Verification items for this drawing (mm, ordinates from the low corner). Coordinates: 2 decimals unless noted, no trailing zeros. Loops run counter-clockwise (first coordinate to the right, second up) from the corner with the lowest first, then second, coordinate; pieces in that order, holes last. Notation, with made-up numbers: (28, -31.75) -> (59, -31.75) arc R15 cw to (59, -20.75) -> close; hole circle Ø1 at (62, 30). An arc over 180 degrees is marked (long way). Write item = value, one per line.
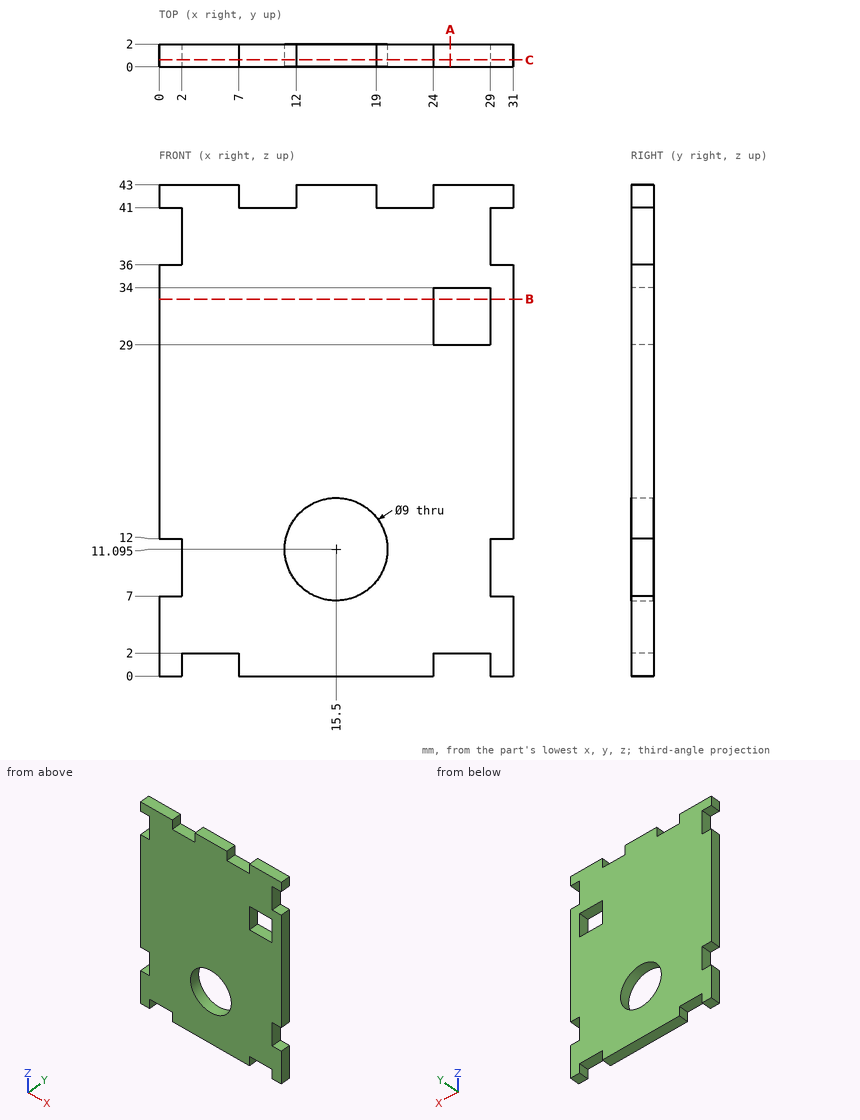
1) Sectioned sample at A-A, the plane x = 25.5. Record the cut outline in (y, z), plus the area to 3 significant figures.
Ans:
outline = (0, 2) -> (2, 2) -> (2, 29) -> (0, 29) -> close; (0, 34) -> (2, 34) -> (2, 43) -> (0, 43) -> close
area = 72.0 mm2
2) Sectioned sample at B-B, the plane z = 33. Record the cut outline in (x, y), plus the area to 3 significant figures.
Ans:
outline = (0, 0) -> (24, 0) -> (24, 2) -> (0, 2) -> close; (29, 0) -> (31, 0) -> (31, 2) -> (29, 2) -> close
area = 52.0 mm2
3) Sectioned sample at C-C, the plane y = 0.6. Count the separate pieces of the cut face and the enclosed holes in it, plus the area to 3 significant figures.
Ans:
separate_pieces = 1
enclosed_holes = 2
area = 1,160 mm2
4) Material ranges on line 1 (Z direction, x = 15.5, y = 1.15) (3 decimals); line 2 (Z direction, x = 26, y = 1.35); line 3 (X direction, y = 0.7, z = 13.5), recorded low to high.
Ans:
line_1 = 0 to 6.595, 15.595 to 43
line_2 = 2 to 29, 34 to 43
line_3 = 0 to 11.7, 19.3 to 31
5) Depth check by flat-ended pin: pin 1 Ø1 at (y, z) = (1, 10.5) entering from -X; pin 2 Ø1 at (y, z) = (1, 24.5) entering from -X; pin 3 Ø1 at (y, z) = (1, 10.5) entering from +X. Enter the tip coordinate at first touch or a pass-through.
Ans:
pin_1 = 2
pin_2 = 0
pin_3 = 29
